Verification items for the finished model (mm, model axes). Face numbers are marked on the shaded views. Give positions to 0.01 mm unless a question says otherwise; leave off trailing zeros. Write each loop counter-clockwise with the first axis right and the second up, starting at its lowest first coordinate (ties: lowest second). Pieces come first, ordered by that corner, then holes. Notation, with made-up numbers: (75, 28) -> (103, 28) arc R25 cw to (103, 49) -> close; hole circle Ø10 at (-3, -24.5). An arc over 180 degrees is marked (long way). Write item = value, one per line.
from build123d import *

# Parameters (mm, degrees)
BOSS_EXTRUDE1_DEPTH   = 30
F_3_0MM_DOWEL_HOLE1_D = 3


with BuildPart() as part:
    # Sketch1 → Boss-Extrude1 (new body)
    with BuildSketch(Plane(origin=(0, 0, 0), x_dir=(0, 0, -1), z_dir=(1, 0, 0))):
        with BuildLine():
            Line((-17.5, 0), (-17.5, 15))
            Line((-17.5, 15), (17.5, 15))
            Line((17.5, 15), (17.5, 0))
            Line((17.5, 0), (12.2, 0))
            ThreePointArc((12.2, 0), (0, 12.2), (-12.2, 0))
            Line((-12.2, 0), (-17.5, 0))
        make_face()
    extrude(amount=BOSS_EXTRUDE1_DEPTH)

    # Ø3.0mm Dowel Hole1 (through all)
    with Locations(Plane(origin=(15, 15, -14.85), x_dir=(0, 0, 1), z_dir=(0, 1, 0))):
        with Locations((0, 0), (29.7, 0)):
            Hole(F_3_0MM_DOWEL_HOLE1_D / 2)


solid = part.part
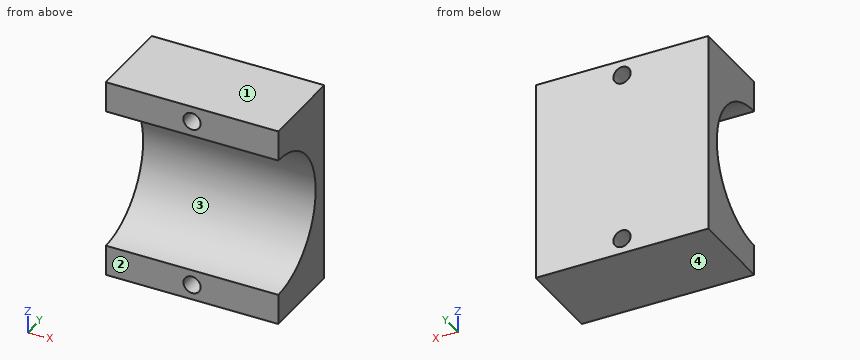
Item 1: Material ranges on line 1 (X direction, y = 9, z = -14.85); line 2 (Z direction, x = 16, y = 4.75); line 3 (Z direction, x = 7, y = 2.5), recorded low to high.
Response values:
line_1 = 0 to 13.5, 16.5 to 30
line_2 = -17.5 to -15.97, -13.73 to -11.24, 11.24 to 13.73, 15.97 to 17.5
line_3 = -17.5 to -11.94, 11.94 to 17.5
Item 2: Sectioned sample at C-C on y = 5. Record the cut outline in (x, z), then the cut area to 3 significant figures.
Response values:
outline = (0, -17.5) -> (30, -17.5) -> (30, -11.13) -> (0, -11.13) -> close; (0, 11.13) -> (30, 11.13) -> (30, 17.5) -> (0, 17.5) -> close; hole circle Ø3 at (15, -14.85); hole circle Ø3 at (15, 14.85)
area = 368 mm^2
Item 3: Sectioned sample at B-B on z = -14.85. Record the cut outline in (x, y), then the cut area to 3 significant figures.
Response values:
outline = (0, 0) -> (13.5, 0) -> (13.5, 15) -> (0, 15) -> close; (16.5, 0) -> (30, 0) -> (30, 15) -> (16.5, 15) -> close
area = 405 mm^2
Item 4: Sectioned sample at D-D on y = 11. Record the cut outline in (x, z).
Response values:
outline = (0, -17.5) -> (30, -17.5) -> (30, -5.28) -> (0, -5.28) -> close; (0, 5.28) -> (30, 5.28) -> (30, 17.5) -> (0, 17.5) -> close; hole circle Ø3 at (15, -14.85); hole circle Ø3 at (15, 14.85)
Item 5: Mould release check, pull along Z, two halves, no side actions. Record for the marked faces 1, 2, 3 and 4: +Z half, -Z half, draft (parallel to the pull), parting line (faces both ways), or undercut.
Response values:
face_1 = +Z half
face_2 = draft
face_3 = undercut
face_4 = -Z half
Item 6: Sectioned sample at A-A on x = 15. Record the cut outline in (y, z).
Response values:
outline = (0, -17.5) -> (15, -17.5) -> (15, -16.35) -> (0, -16.35) -> close; (0, -13.35) -> (15, -13.35) -> (15, 13.35) -> (0, 13.35) -> (0, 12.2) arc R12.2 cw to (0, -12.2) -> close; (0, 16.35) -> (15, 16.35) -> (15, 17.5) -> (0, 17.5) -> close
